Check sheet for the modelled part. Datum: model origin and axes. Units: mm. A direction names the side the tool comes from. Round coordinates to 2 decimals unless told otherwise and drop trailing zeros. Write each loop counter-clockwise with the first axis right and the second up, starting at its lowest first coordinate (ties: lowest second). Pieces come first, ordered by that corner, then holes. Notation, with made-up numbers: (40.5, 52) -> (76.5, 52) arc R20 ccw to (76.5, 84) -> close; hole circle Ø6 at (6, -2.5). An arc over 180 degrees is marked (long way). One line per item, written item: value.
from build123d import *

# Parameters (mm, degrees)
BOSS_EXTRUDE2_DEPTH     = 24
CUT_EXTRUDE1_DEPTH      = 82.49233092751734
CUT_EXTRUDE1_DEPTH_BACK = 82.49233092751734
SKETCH17_R              = 1.9999999999999996
SKETCH17_R_2            = 1.9999999999999962
F_3_0MM_DOWEL_HOLE1_D   = 3
SKETCH22_R              = 5.000000000000001
SKETCH22_R_2            = 4.9999999999999964
CUT_EXTRUDE2_DEPTH      = 1.5
CUT_EXTRUDE3_DEPTH      = 68.21792915584354
CUT_EXTRUDE3_DEPTH_BACK = 68.21792915584354
SKETCH23_W              = 9.949874371066619
SKETCH23_H              = 10
FILLET1_R               = 1


with BuildPart() as part:
    # 3DSketch1 → Boss-Extrude2 (new body)
    with BuildSketch(Plane(origin=(0, 0, 0), x_dir=(0.9998052854172774, 0.01973299905428837, 0), z_dir=(-3e-17, -8.8e-16, 1))):
        Polygon((0, 0), (17.496592494802357, -0.34532748345004655), (17.832053478725257, 16.65136236864367), (58.82407018083363, 15.842309407417849), (58.48860919691073, -1.1543804446758696), (75.98520169171307, -1.499707928125916), (76.0148011902945, 2.2e-16), (60.01791662361808, 0.3157279848686118), (60.353377607540985, 17.312417836962325), (16.361945049180772, 18.180669795351015), (16.02648406525787, 1.1839799432573024), (0.02959949858143255, 1.4997079281259162), align=None)
    extrude(amount=BOSS_EXTRUDE2_DEPTH)

    # Sketch17 → Cut-Extrude1 (cut, two sides: drawn at the far end of the back side and taken through both)
    with BuildSketch(Plane(origin=(0, 1.5, 0), x_dir=(1, 0, 0), z_dir=(0, 1, 0)).offset(-CUT_EXTRUDE1_DEPTH_BACK)):
        with Locations(Location((8, -12.000000000000002, 0), (0, 0, 270))):
            Circle(SKETCH17_R)
        with Locations(Location((68, -12.000000000000002, 0), (0, 0, 270))):
            Circle(SKETCH17_R_2)
    extrude(amount=CUT_EXTRUDE1_DEPTH + CUT_EXTRUDE1_DEPTH_BACK, mode=Mode.SUBTRACT)

    # Ø3.0mm Dowel Hole1 (through all)
    with Locations(Plane(origin=(0, 18.5, 0), x_dir=(1, 0, 0), z_dir=(0, 1, 0))):
        with Locations((28.5, -12), (47.5, -12), (38, -19.8), (38, -4.2)):
            Hole(F_3_0MM_DOWEL_HOLE1_D / 2)

    # Sketch22 → Cut-Extrude2 (cut)
    with BuildSketch(Plane(origin=(0, 1.5, 0), x_dir=(1, 0, 0), z_dir=(0, 1, 0))):
        with Locations((17.999999999997943, -12.000000000000927)):
            Circle(SKETCH22_R)
        with Locations((58.00000000000207, -12.000000000000927)):
            Circle(SKETCH22_R_2)
    extrude(amount=-CUT_EXTRUDE2_DEPTH, mode=Mode.SUBTRACT)

    # Sketch23 → Cut-Extrude3 (cut, two sides: drawn at the far end of the back side and taken through both)
    with BuildSketch(Plane.ZY.offset(-16).offset(-CUT_EXTRUDE3_DEPTH_BACK)):
        with Locations((12.000000000000927, 6.5)):
            Rectangle(SKETCH23_W, SKETCH23_H)
    extrude(amount=CUT_EXTRUDE3_DEPTH + CUT_EXTRUDE3_DEPTH_BACK, mode=Mode.SUBTRACT)

    # Fillet1
    fillet1_edges = [part.edges().sort_by_distance(p)[0] for p in [
        (17.500000000000004, -3.09e-15, 3.5125314072338187),
        (17.500000000000004, -1.8e-14, 20.487468592767108),
        (58.50000000000001, -3.09e-15, 3.5125314072338214),
        (58.50000000000001, -1.8e-14, 20.487468592767108),
        (15.999999999999998, 18.49999999999999, 12.000000000000016),
        (60.000000000000014, 18.49999999999999, 12.000000000000018),
        (60.00000000000001, 1.49999999999998, 20.48746859276712),
        (60.00000000000001, 1.499999999999995, 3.512531407233811),
        (15.999999999999998, 1.4999999999999825, 20.48746859276712),
        (15.999999999999998, 1.4999999999999973, 3.5125314072338103),
    ]]
    fillet(fillet1_edges, radius=FILLET1_R)


solid = part.part
Item 1: Sectioned sample at A-A (x = 14). Enter the section's corners in (y, z).
Result set:
outline: (0, 0) -> (1.5, 0) -> (1.5, 9) -> (0, 9) -> close; (0, 15) -> (1.5, 15) -> (1.5, 24) -> (0, 24) -> close
Item 2: Sectioned sample at D-D (x = 38). Enter the section's corners in (y, z), then the cut area to 3 significant figures.
Result set:
outline: (17, 0) -> (18.5, 0) -> (18.5, 2.7) -> (17, 2.7) -> close; (17, 5.7) -> (18.5, 5.7) -> (18.5, 18.3) -> (17, 18.3) -> close; (17, 21.3) -> (18.5, 21.3) -> (18.5, 24) -> (17, 24) -> close
area: 27.0 mm^2
Item 3: Material ranges on line 1 along X through (y, z) = (1.15, 12); line 2 along Z through (x, y) = (38, 18.05); line 3 along Z through (x, y) = (8, 1.2), recorded low to high.
Result set:
line 1: 0 to 6, 10 to 13, 63 to 66, 70 to 76
line 2: 0 to 2.7, 5.7 to 18.3, 21.3 to 24
line 3: 0 to 10, 14 to 24
Item 4: Depth check by flat-ended pin: pin 1 (2.5 mm diameter, centred on x = 38, z = 19.8, fed in from +Y); pin 2 (8 mm diameter, centred on y = 6, z = 3.5, fed in from +X); pin 3 (5 mm diameter, centred on y = 13, z = 16.5, fed in from -X); pin 4 (0.8 mm diameter, centred on x = 59, z = 13, fed in from -Y). Enter the tip coordinate at first touch or a pass-through.
Result set:
pin 1: through
pin 2: x = 60.13
pin 3: x = 16
pin 4: y = 11.5
Item 5: Tool access check on faces 1 (the flat face through (17, 6, 16.975)), 2 (the flat face through (16, 12, 12)), 3 (the cylindrical face through (13, 1, 12)), 4 (the cylindrical face through (30, 18, 12)). Record the directions out of +Z, -Z, +X, -X, +Y, -Y that give a thin tool (end or side, any length) a straight path to the whole face; none if there is none.
Result set:
face 1: +X, -X
face 2: +Z, -Z, -X, +Y
face 3: -Y
face 4: +Y, -Y
Item 6: Release check for a two-part mould opening along Z. For faces 5 (the flat face through (17, 11.5, 12)), 6 (the flat face through (40.3, 17.2, 24)), 7 (the flat face through (58.5, 13, 12)), 8 (the flat face through (40.3, 17.2, 0)) record: pulls with the +Z half, pulls with the -Z half, needs draft (parallel to the pull), parting line crosses it, or undercut.
Result set:
face 5: undercut
face 6: pulls with the +Z half
face 7: needs draft
face 8: pulls with the -Z half
Item 7: Sectioned sample at B-B (z = 9). Enter the section's corners in (x, y).
Result set:
outline: (0, 0) -> (14, 0) -> (14, 1.5) -> (0, 1.5) -> close; (16, 11.5) -> (17.5, 11.5) -> (17.5, 17) -> (58.5, 17) -> (58.5, 11.5) -> (60, 11.5) -> (60, 17.5) arc R1 ccw to (59, 18.5) -> (17, 18.5) arc R1 ccw to (16, 17.5) -> close; (62, 0) -> (76, 0) -> (76, 1.5) -> (62, 1.5) -> close
Item 8: Sectioned sample at C-C (y = 10.5). Enter the section's corners in (x, z), then the cut area to 3 significant figures.
Result set:
outline: (16, 0) -> (17.5, 0) -> (17.5, 7.03) -> (16, 7.03) -> close; (16, 16.97) -> (17.5, 16.97) -> (17.5, 24) -> (16, 24) -> close; (58.5, 0) -> (60, 0) -> (60, 7.03) -> (58.5, 7.03) -> close; (58.5, 16.97) -> (60, 16.97) -> (60, 24) -> (58.5, 24) -> close
area: 42.2 mm^2
